from build123d import *

# Parameters (mm, degrees)
F1_DEPTH = 1.5
F2_R     = 2.1
F2_R_2   = 0.6
F3_DEPTH = 1.501


# Not quite as in the source:
# - a feature names something its author has since deleted; it is built from what else it names


with BuildPart() as f1:
    # F0 (on Top) → F1 (new body)
    with BuildSketch(Plane.XY):
        with BuildLine():
            Line((83, -42), (-83, -42))
            Line((-83, -42), (-83, -54))
            ThreePointArc((-83, -54), (-82.7071067812, -54.7071067812), (-82, -55))
            Line((-82, -55), (82, -55))
            ThreePointArc((82, -55), (82.7071067812, -54.7071067812), (83, -54))
            Line((83, -54), (83, -42))
        make_face()
        Polygon((89.5, 42), (-89.5, 42), (-89.5, -42), (-83, -42), (83, -42), (89.5, -42), align=None)
    extrude(amount=F1_DEPTH)

    # F2 (on face) → F3 (cut, through all)
    with BuildSketch(Plane.XY.offset(1.5)):
        with Locations((-85.5, -38)):
            Circle(F2_R)
        with Locations((-85.5, 23)):
            Circle(F2_R)
        Polygon((-89.5, 42), (-89.5, 37.5), (-85, 42), align=None)
        with Locations((85.5, -38)):
            Circle(F2_R)
        Polygon((89.5, 42), (85, 42), (89.5, 37.5), align=None)
        with Locations((85.5, 23)):
            Circle(F2_R)
        with Locations((-58, -35)):
            Circle(F2_R_2)
        with Locations((-58, -30)):
            Circle(F2_R_2)
        with Locations((-58, -25)):
            Circle(F2_R_2)
        with Locations((-58, -20)):
            Circle(F2_R_2)
        with Locations((-58, -15)):
            Circle(F2_R_2)
        with Locations((-58, -10)):
            Circle(F2_R_2)
        with Locations((-58, -5)):
            Circle(F2_R_2)
        with Locations((-58, 0)):
            Circle(F2_R_2)
        with Locations((-58, 5)):
            Circle(F2_R_2)
        with Locations((-58, 10)):
            Circle(F2_R_2)
        with Locations((-18, 10)):
            Circle(F2_R_2)
        with Locations((-18, 5)):
            Circle(F2_R_2)
        with Locations((-18, 0)):
            Circle(F2_R_2)
        with Locations((-18, -5)):
            Circle(F2_R_2)
        with Locations((-18, -10)):
            Circle(F2_R_2)
        with Locations((-18, -15)):
            Circle(F2_R_2)
        with Locations((-18, -20)):
            Circle(F2_R_2)
        with Locations((-18, -25)):
            Circle(F2_R_2)
        with Locations((-18, -30)):
            Circle(F2_R_2)
        with Locations((-18, -35)):
            Circle(F2_R_2)
        with Locations((22, -35)):
            Circle(F2_R_2)
        with Locations((22, -30)):
            Circle(F2_R_2)
        with Locations((22, -25)):
            Circle(F2_R_2)
        with Locations((22, -20)):
            Circle(F2_R_2)
        with Locations((22, -15)):
            Circle(F2_R_2)
        with Locations((22, -10)):
            Circle(F2_R_2)
        with Locations((22, -5)):
            Circle(F2_R_2)
        with Locations((22, 0)):
            Circle(F2_R_2)
        with Locations((22, 5)):
            Circle(F2_R_2)
        with Locations((22, 10)):
            Circle(F2_R_2)
        with Locations((62, 10)):
            Circle(F2_R_2)
        with Locations((62, 5)):
            Circle(F2_R_2)
        with Locations((62, 0)):
            Circle(F2_R_2)
        with Locations((62, -5)):
            Circle(F2_R_2)
        with Locations((62, -10)):
            Circle(F2_R_2)
        with Locations((62, -15)):
            Circle(F2_R_2)
        with Locations((62, -20)):
            Circle(F2_R_2)
        with Locations((62, -25)):
            Circle(F2_R_2)
        with Locations((62, -30)):
            Circle(F2_R_2)
        with Locations((62, -35)):
            Circle(F2_R_2)
    extrude(amount=-F3_DEPTH, mode=Mode.SUBTRACT)


solid = f1.part
Here's how the part is built. I have some questions about the finished solid (model axes, mm). Coordinates: 2 decimals unless noted, no trailing zeros. Write each loop counter-clockwise with the first axis right and the second up, starting at its lowest first coordinate (ties: lowest second). Pieces come first, ordered by that corner, then holes.
Item 1: I want a section at A-A on y = -38. Write out the boundary of the cut face in (x, z).
Item 2: I want a section at B-B on z = 0.7. Count the separate pieces of the cut face and the enclosed holes in it, and give its area (3 significant figures).
Item 3: Will this pin go through, and if not, where does the flat tip stop? pin 1 (6 mm diameter, centred on x = 28.5, y = 18, fed in from -Z).
Item 4: If we mould it in two halves opening along X, with no side actions, what happens to faces 1 (the flat face through (87, 40, 1)), 2 (the cylindrical face through (-87.6, 23.09, 0.76)), 3 (the flat face through (-1, -6, 1.5))? For each: +X half, -X half, draft (parallel to the pull), parting line (faces both ways), or undercut.
Item 5: If I drill on line 1 (Y direction, x = -85.5, z = 0.9); line 2 (X direction, y = -39.5, z = 0.6); line 3 (X direction, y = 23.5, z = 0.7), over which ranges is the centre line in solid material (lowest first)?
Findings below:
1. outline: (-89.5, 0) - (-87.6, 0) - (-87.6, 1.5) - (-89.5, 1.5) - close; (-83.4, 0) - (83.4, 0) - (83.4, 1.5) - (-83.4, 1.5) - close; (87.6, 0) - (89.5, 0) - (89.5, 1.5) - (87.6, 1.5) - close
2. separate pieces: 1
2. enclosed holes: 44
2. area: 17,100 mm2
3. pin 1: stops at z = 0
4. face 1: +X half
4. face 2: undercut
4. face 3: draft
5. line 1: y = -42 to -40.1, -35.9 to 20.9, 25.1 to 41.5
5. line 2: x = -89.5 to -86.97, -84.03 to 84.03, 86.97 to 89.5
5. line 3: x = -89.5 to -87.54, -83.46 to 83.46, 87.54 to 89.5
